CAD build for the part. Positions are in the model's coordinates, mm. Give positions to 0.01 mm unless a question says otherwise; leave off trailing zeros. Write each loop counter-clockwise with the first axis right and the second up, starting at its lowest first coordinate (ties: lowest second). Pieces come first, ordered by that corner, then holes. Notation, with made-up numbers: (-8, 55) - (4, 55) arc R18 ccw to (4, 61) - close; hole circle Ø7 at (24.5, 10.25). An arc over 180 degrees is marked (long way). Answer as a JSON object with one key per item and string values.
from build123d import *

# Parameters (mm, degrees)
SKETCH1_R           = 350
SKETCH1_R_2         = 15
BOSS_EXTRUDE1_DEPTH = 100
SKETCH2_W           = 100
SKETCH2_H           = 100
CUT_EXTRUDE1_DEPTH  = 500
SKETCH3_W           = 500
SKETCH3_H           = 400
SKETCH3_W_2         = 490
SKETCH3_H_2         = 390
CUT_EXTRUDE2_DEPTH  = 1
SKETCH4_R           = 25
SKETCH4_R_2         = 20
CUT_EXTRUDE3_DEPTH  = 10


with BuildPart() as part:
    # Sketch1 → Boss-Extrude1 (new body)
    with BuildSketch(Plane.XY):
        Circle(SKETCH1_R)
        Circle(SKETCH1_R_2, mode=Mode.SUBTRACT)
    extrude(amount=BOSS_EXTRUDE1_DEPTH)

    # Sketch2 → Cut-Extrude1 (cut, symmetric)
    with BuildSketch(Plane(origin=(0, 0, 0), x_dir=(0, 0, -1), z_dir=(1, 0, 0))):
        Polygon((-100, 7), (-83, 7), (-83, 12), (-75, 12), (-75, -12), (-83, -12), (-83, -7), (-100, -7), align=None)
        Polygon((-100, -77), (-100, -63), (-83, -63), (-83, -58), (-75, -58), (-75, -82), (-83, -82), (-83, -77), align=None)
        Polygon((-100, -147), (-100, -133), (-83, -133), (-83, -128), (-75, -128), (-75, -152), (-83, -152), (-83, -147), align=None)
        Polygon((-100, -217), (-100, -203), (-83, -203), (-83, -198), (-75, -198), (-75, -222), (-83, -222), (-83, -217), align=None)
        with Locations((-50, -300)):
            Rectangle(SKETCH2_W, SKETCH2_H)
        Polygon((-100, 63), (-100, 77), (-83, 77), (-83, 82), (-75, 82), (-75, 58), (-83, 58), (-83, 63), align=None)
        with Locations((-50, 300)):
            Rectangle(SKETCH2_W, SKETCH2_H)
        Polygon((-100, 133), (-100, 147), (-83, 147), (-83, 152), (-75, 152), (-75, 128), (-83, 128), (-83, 133), align=None)
        Polygon((-100, 203), (-100, 217), (-83, 217), (-83, 222), (-75, 222), (-75, 198), (-83, 198), (-83, 203), align=None)
    extrude(amount=CUT_EXTRUDE1_DEPTH, both=True, mode=Mode.SUBTRACT)

    # Sketch3 → Cut-Extrude2 (cut)
    with BuildSketch(Plane.XY.offset(100)):
        with Locations((49.34, 6.2164)):
            Rectangle(SKETCH3_W, SKETCH3_H)
        with Locations((49.34, 6.2164)):
            Rectangle(SKETCH3_W_2, SKETCH3_H_2, mode=Mode.SUBTRACT)
    extrude(amount=-CUT_EXTRUDE2_DEPTH, mode=Mode.SUBTRACT)

    # Sketch4 → Cut-Extrude3 (cut)
    with BuildSketch(Plane.XZ.offset(-250)):
        with Locations(Location((0, 50, 0), (0, 0, 270))):
            Circle(SKETCH4_R)
        with Locations(Location((144.948974278, 50, 0), (0, 0, 270))):
            Circle(SKETCH4_R_2)
        with Locations(Location((-144.948974278, 50.764190285, 0), (0, 0, 270))):
            Circle(SKETCH4_R_2)
    extrude(amount=CUT_EXTRUDE3_DEPTH, mode=Mode.SUBTRACT)


solid = part.part
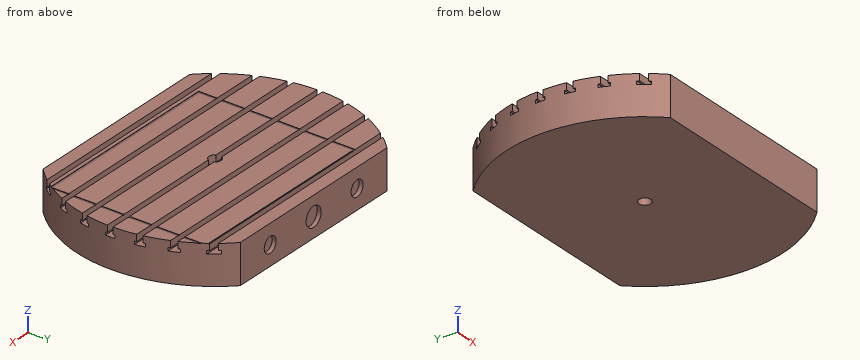
(1) Flat gauge pins, fed straight in: P1, Ø0.5, axis at y = -47, z = 99.5, coming from the +X side; P2, Ø1, axis at x = 52.5, y = 139.5, coming from the +Z side; P3, Ø18.5, axis at x = 257, z = 91.5, coming from the +Y side. Where does each tip first touch, or does it go through?
Answer key:
{"P1": "stops at x = 346.86", "P2": "stops at z = 75", "P3": "stops at y = 247.22"}
(2) Saw through at A-A, the plane y = 0. Give the cut face in (x, z).
Answer key:
{"outline": "(-350, 0) - (-15, 0) - (-15, 75) - (-350, 75) - close; (15, 0) - (350, 0) - (350, 75) - (15, 75) - close"}
(3) Saw through at B-B, the plane z = 43. Give the cut face in (x, y).
Answer key:
{"outline": "(-244.95, -250) - (244.95, -250) arc R350 ccw to (244.95, 250) - (163.68, 250) - (163.68, 240) - (126.21, 240) - (126.21, 250) - (24, 250) - (24, 240) - (-24, 240) - (-24, 250) - (-126.52, 250) - (-126.52, 240) - (-163.38, 240) - (-163.38, 250) - (-244.95, 250) arc R350 ccw to start; hole circle Ø30 at (0, 0)"}
(4) Probe L1, parallel to Z at x = 205.5, y = 148; L2, parallel to X at y = -0.5, z = 60.5; L3, parallel to Y at x = 0, z = 35.5. List the from-to ranges inside material, lowest first. Write a range as [from, to].
Answer key:
{"L1": "z = [0, 75], [83, 100]", "L2": "x = [-350, -14.99], [14.99, 350]", "L3": "y = [-250, -15], [15, 240]"}
(5) Saw through at C-C, the plane y = -99.5. Give the cut face in (x, z).
Answer key:
{"outline": "(-335.56, 0) - (335.56, 0) - (335.56, 100) - (299.34, 100) - (299.34, 99) - (294.34, 99) - (294.34, 100) - (-195.66, 100) - (-195.66, 99) - (-200.66, 99) - (-200.66, 100) - (-335.56, 100) - close"}
